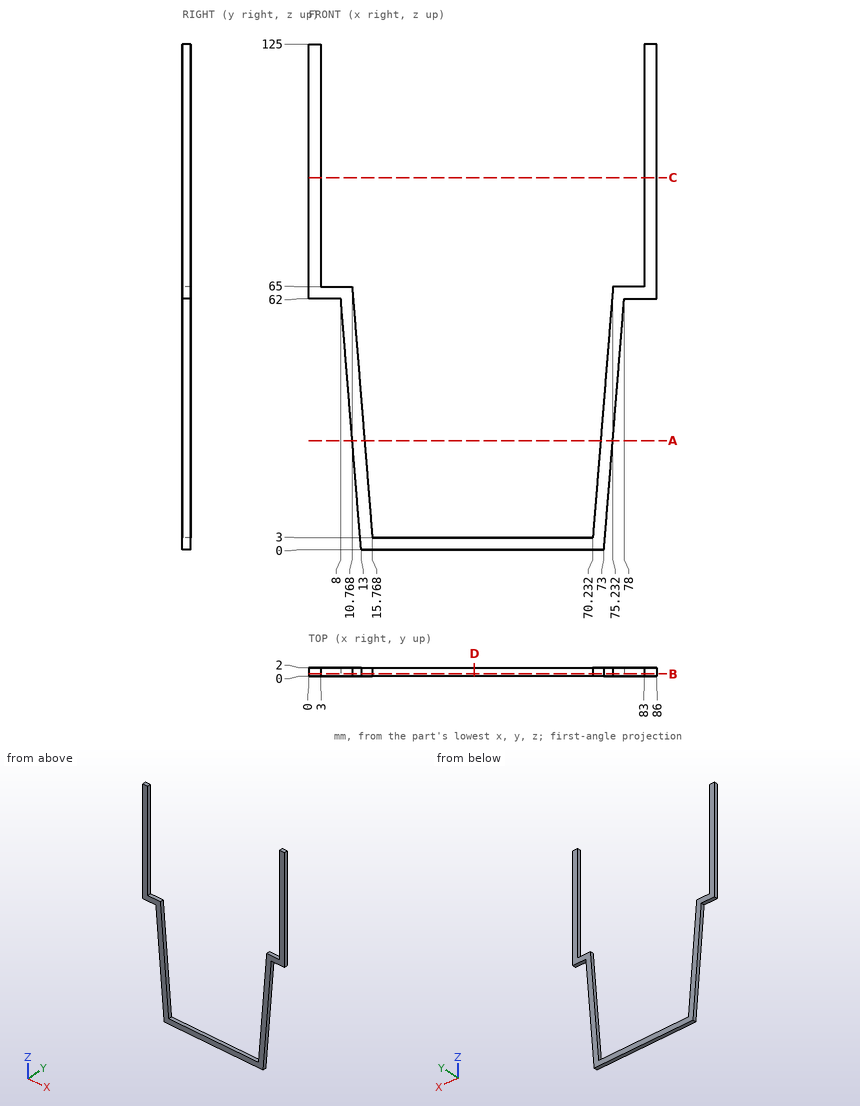
The drawing under review shows one solid part. Ordinate dimensions are in mm from its lowest x, y, z. Coordinates: 2 decimals unless noted, no trailing zeros. Write each loop counter-clockwise with the first axis right and the second up, starting at its lowest first coordinate (ties: lowest second). Pieces come first, ordered by that corner, then holes. Notation, with made-up numbers: (-17, -29.75) - (28, -29.75) arc R12 ccw to (28, -8.75) - close; hole circle Ø11 at (67.5, 49.5). An arc over 180 degrees is marked (long way). Answer as CSV lines item,"result".
(1) We need section B-B (y = 0.55). Give the boundary of the cut face in (x, z), plus the area to 3 significant figures.
Data:
outline,"(0, 62) - (8, 62) - (13, 0) - (73, 0) - (78, 62) - (86, 62) - (86, 125) - (83, 125) - (83, 65) - (75.23, 65) - (70.23, 3) - (15.77, 3) - (10.77, 65) - (3, 65) - (3, 125) - (0, 125) - close"
area,"961 mm2"
(2) We need section A-A (z = 27). Give the boundary of the cut face in (x, y).
Data:
outline,"(10.82, 0) - (13.83, 0) - (13.83, 2) - (10.82, 2) - close; (72.17, 0) - (75.18, 0) - (75.18, 2) - (72.17, 2) - close"
(3) Clearance check with flat-ended pins moving along their axes: pin 1 Ø0.6 at (x, y) = (7, 1) entering from +Z; pin 2 Ø1 at (x, y) = (48, 1) entering from +Z. State where each tip first meets the part, or that it passes through.
Data:
pin 1,"stops at z = 65"
pin 2,"stops at z = 3"
(4) We need section C-C (z = 92). Give the boundary of the cut face in (x, y).
Data:
outline,"(0, 0) - (3, 0) - (3, 2) - (0, 2) - close; (83, 0) - (86, 0) - (86, 2) - (83, 2) - close"
(5) We need section D-D (x = 41). Give the boundary of the cut face in (y, z).
Data:
outline,"(0, 0) - (2, 0) - (2, 3) - (0, 3) - close"
(6) For line 1 along X through (y, z) = (1, 84); line 2 along Z through (x, y) = (38.5, 0.8); line 3 along X through (y, z) = (1.3, 45), list the stretches that pass through material, from the lowest coordinate up. Write a range as [from, to].
Data:
line 1,"x = [0, 3], [83, 86]"
line 2,"z = [0, 3]"
line 3,"x = [9.37, 12.38], [73.62, 76.63]"
